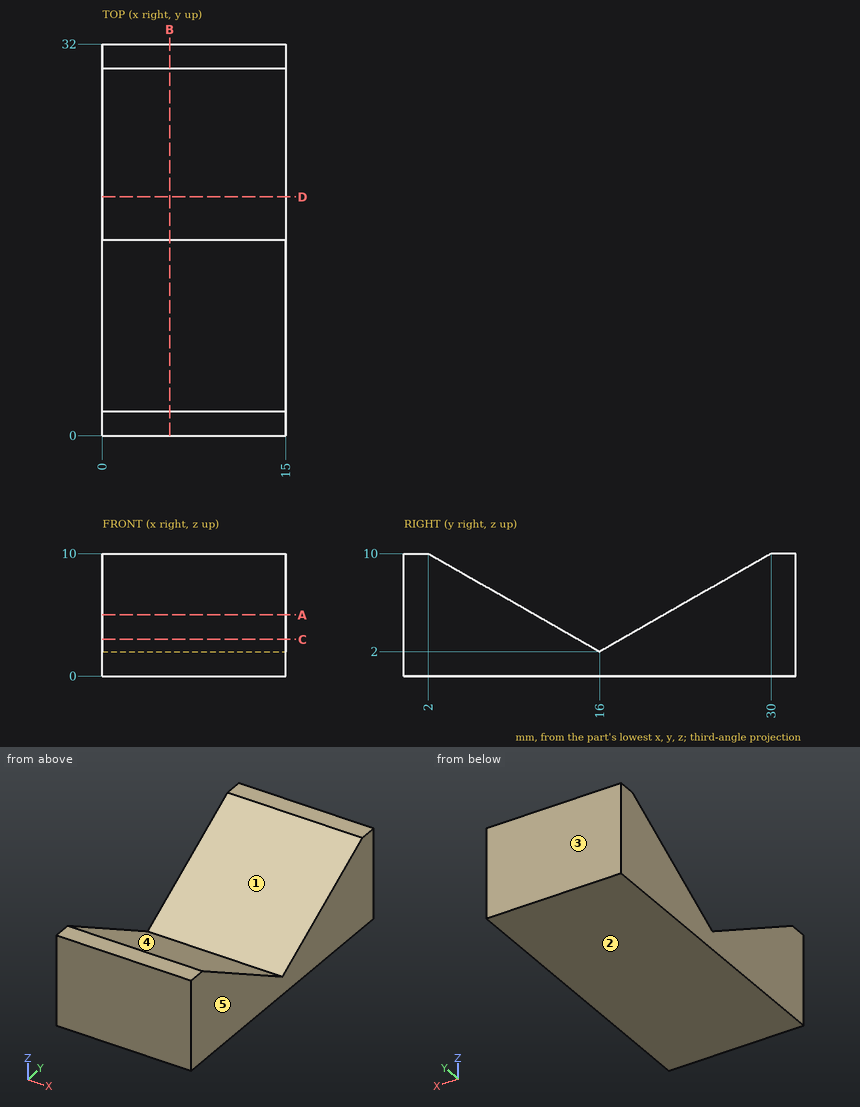
The figure shows three views and two pictorial views of one solid part (mm, origin at its lowest corner). Answer the questions. A direction names the side the tool comes from. Give positions to 0.01 mm unless a question says otherwise; leave off trailing zeros. Order: outer loops, then holes, each group sorted by start corner. A loop starts at its lowest first (then second) coordinate and runs counter-clockwise, first axis right, second up. Notation, with made-up numbers: M 42.25,15.5 L 71.25,15.5 A26 ccw 71.25,45.5 Z; hole C 20.25,69 d6. An arc over 180 degrees is marked long. Return JSON: item names as keys, results as strings.
Q1. The mould has two halves that part along Y. Classify the marked faces 3, 4 and 5: pulls with the +Y half, pulls with the -Y half, needs draft (parallel to the pull), parting line crosses it, or undercut.
Answer below:
{"face 3": "pulls with the +Y half", "face 4": "undercut", "face 5": "needs draft"}
Q2. Find section C-C, the plane z = 3. Write down the section's boundary in (x, y).
Answer below:
{"outline": "M 0,0 L 15,0 L 15,14.25 L 0,14.25 Z; M 0,17.75 L 15,17.75 L 15,32 L 0,32 Z"}
Q3. Which of the six approach directions +Z, -Z, +X, -X, +Y, -Y give full straight-line access (tool end or side, diameter ignored) to the marked faces 1 and 2?
Answer below:
{"face 1": "+Z, +X, -X", "face 2": "-Z, +X, -X, +Y, -Y"}
Q4. Find the intervals of material crossed by line 1 along Y through (x, z) = (4.75, 2.5) (3 decimals); line 2 along Y through (x, z) = (7.5, 9.25); line 3 along Z through (x, y) = (1.5, 6.5), in increasing order. Write a range as [from, to].
Answer below:
{"line 1": "y = [0, 15.125], [16.875, 32]", "line 2": "y = [0, 3.31], [28.69, 32]", "line 3": "z = [0, 7.43]"}
Q5. Find section D-D, the plane y = 19.5. Write down the section's boundary in (x, z).
Answer below:
{"outline": "M 0,0 L 15,0 L 15,4 L 0,4 Z"}
Q6. Each of these flat-tipped pins is pushed along its axis until it touches: pin 1 (4 mm diameter, centred on x = 8.5, z = 6.5, fed in from -Y); pin 2 (1.5 mm diameter, centred on x = 11.5, y = 14, fed in from +Z); pin 3 (1 mm diameter, centred on x = 4.5, y = 12, fed in from +Z). Where does it stop, or does it pass through?
Answer below:
{"pin 1": "stops at y = 0", "pin 2": "stops at z = 3.57", "pin 3": "stops at z = 4.57"}
Q7. Find section B-B, the plane x = 5.5. Write down the section's boundary in (y, z).
Answer below:
{"outline": "M 0,0 L 32,0 L 32,10 L 30,10 L 16,2 L 2,10 L 0,10 Z"}
Q8. Find section A-A, the plane z = 5. Write down the section's boundary in (x, y).
Answer below:
{"outline": "M 0,0 L 15,0 L 15,10.75 L 0,10.75 Z; M 0,21.25 L 15,21.25 L 15,32 L 0,32 Z"}
